Could you check a few things on this model? Use its own coordinates, in mm. A direction names the side the tool comes from. Coordinates: 2 decimals unless noted, no trailing zeros. Order: outer loops, then holes, each group sorted by start corner. A loop starts at its lowest first (then second) coordinate and runs counter-clockwise, first axis right, second up. Notation, with made-up numbers: (-13, -16) - (28, -16) arc R26 ccw to (28, 10) - close; hole circle Ø10 at (36, 26). An arc over 180 degrees is marked (long way). Answer as CSV lines item,"result". Start each with the question number.
1. I need wall thicknesses on probe 1 along X at (y, z) = (-20, 2.4); probe 2 along Y at (x, z) = (12.7, 2.05) (3 decimals); probe 3 along Y at (x, z) = (11, 0.4) (3 decimals). Which ranges of each line are inside material? Lowest first, please.
2. I want a section at C-C, the plane x = 28. List the corners of the cut face in (y, z) for me, and give its area (3 significant figures).
3. Thinking about a two-plate mould opening in Y: for faces 1 (the face through (-33.94, -21.77, 2.96)), 2 (the face through (31.242, 0, 3)), 3 (the face through (-25.4, -21, 3)), which applies, released by +Y, released by -Y, zero draft, split by the parting line, or undercut?
4. I want a section at D-D, the plane y = 0. List the corners of the cut face in (x, z) for me.
5. I want a section at A-A, the plane x = -12.7. List the corners of the cut face in (y, z) for me (3 decimals).
6. For faces 4 (the face through (33.96, 21.75, 2.96)), 5 (the face through (0, 5, 0)), 6 (the face through (31.242, -21, 3)), 7 (the face through (-25.4, 0, 3)), 8 (the face through (-28, 19.05, 3)), which set-ups out of +Z, -Z, +X, -X, +Y, -Y let a thin tool reach every point of the face, with its end or its side?
7. I want a section at B-B, the plane y = 12.7. List the corners of the cut face in (x, z) for me, and give its area (3 significant figures).
8. For pin 1 (5 mm diameter, centred on x = -26.5, y = -3.5, fed in from -Z); pin 2 (1.8 mm diameter, centred on x = -29, z = 3.5, fed in from +Y); pin 3 (3 mm diameter, centred on x = -28, z = 3.5, fed in from -Y), each with a flat end and sliding along its axis, tell me the tip position at first contact or that it passes through.
from build123d import *

# Parameters (mm, degrees)
SKETCH1_W           = 5.842
SKETCH1_H           = 12.7
BOSS_EXTRUDE1_DEPTH = 5.842
FILLET1_R           = 1.5875
SKETCH3_R           = 2.38125
CUT_EXTRUDE2_DEPTH  = 42.383686134


with BuildPart() as part:
    # Sketch1 → Boss-Extrude1 (new body)
    with BuildSketch(Plane.XY):
        Polygon((-25.4, -22.225), (25.4, -22.225), (25.4, -19.05), (31.242, -19.05), (31.242, -22.225), (34.417, -22.225), (34.417, 22.225), (31.242, 22.225), (31.242, 19.05), (25.4, 19.05), (25.4, 22.225), (-25.4, 22.225), (-25.4, 19.05), (-31.242, 19.05), (-31.242, 22.225), (-34.417, 22.225), (-34.417, -22.225), (-31.242, -22.225), (-31.242, -19.05), (-25.4, -19.05), align=None)
        with Locations((28.321, 0)):
            Rectangle(SKETCH1_W, SKETCH1_H, mode=Mode.SUBTRACT)
        with Locations((-28.321, 0)):
            Rectangle(SKETCH1_W, SKETCH1_H, mode=Mode.SUBTRACT)
    extrude(amount=BOSS_EXTRUDE1_DEPTH)

    # Fillet1
    fillet1_edges = [part.edges().sort_by_distance(p)[0] for p in [
        (34.417, 22.225, 2.921),
        (34.417, -22.225, 2.921),
        (-34.417, -22.225, 2.921),
        (-34.417, 22.225, 2.921),
    ]]
    fillet(fillet1_edges, radius=FILLET1_R)

    # Sketch3 → Cut-Extrude2 (cut, through all)
    with BuildSketch(Plane.XY.offset(5.842)):
        Circle(SKETCH3_R)
        with Locations((-12.7, 12.7)):
            Circle(SKETCH3_R)
        with Locations(Location((-12.7, -12.7, 0), (0, 0, 180))):
            Circle(SKETCH3_R)
        with Locations((12.7, -12.7)):
            Circle(SKETCH3_R)
        with Locations(Location((12.7, 12.7, 0), (0, 0, 180))):
            Circle(SKETCH3_R)
    extrude(amount=-CUT_EXTRUDE2_DEPTH, mode=Mode.SUBTRACT)


solid = part.part
Solved:
1,probe 1,"x = -34.42 to -31.24, -25.4 to 25.4, 31.24 to 34.42"
1,probe 2,"y = -22.225 to -15.081, -10.319 to 10.319, 15.081 to 22.225"
1,probe 3,"y = -22.225 to -14.367, -11.033 to 11.033, 14.367 to 22.225"
2,outline,"(-19.05, 0) - (-6.35, 0) - (-6.35, 5.84) - (-19.05, 5.84) - close; (6.35, 0) - (19.05, 0) - (19.05, 5.84) - (6.35, 5.84) - close"
2,area,"148 mm2"
3,face 1,"released by -Y"
3,face 2,"undercut"
3,face 3,"zero draft"
4,outline,"(-34.42, 0) - (-31.24, 0) - (-31.24, 5.84) - (-34.42, 5.84) - close; (-25.4, 0) - (-2.38, 0) - (-2.38, 5.84) - (-25.4, 5.84) - close; (2.38, 0) - (25.4, 0) - (25.4, 5.84) - (2.38, 5.84) - close; (31.24, 0) - (34.42, 0) - (34.42, 5.84) - (31.24, 5.84) - close"
5,outline,"(-22.225, 0) - (-15.081, 0) - (-15.081, 5.842) - (-22.225, 5.842) - close; (-10.319, 0) - (10.319, 0) - (10.319, 5.842) - (-10.319, 5.842) - close; (15.081, 0) - (22.225, 0) - (22.225, 5.842) - (15.081, 5.842) - close"
6,face 4,"+Z, -Z, +X, +Y"
6,face 5,"-Z, +X, -X, +Y, -Y"
6,face 6,"+Z, -Z, -Y"
6,face 7,"+Z, -Z"
6,face 8,"+Z, -Z, +Y"
7,outline,"(-34.42, 0) - (-15.08, 0) - (-15.08, 5.84) - (-34.42, 5.84) - close; (-10.32, 0) - (10.32, 0) - (10.32, 5.84) - (-10.32, 5.84) - close; (15.08, 0) - (34.42, 0) - (34.42, 5.84) - (15.08, 5.84) - close"
7,area,"346 mm2"
8,pin 1,"stops at z = 0"
8,pin 2,"stops at y = 19.05"
8,pin 3,"stops at y = -19.05"
